from build123d import *

# Parameters (mm, degrees)
MODEL_R             = 1.2065
BOSS_EXTRUDE1_DEPTH = 6.6


with BuildPart() as part:
    # Model → Boss-Extrude1 (new body)
    with BuildSketch(Plane.XY):
        with BuildLine():
            Line((-38.1, -33.25), (-38.1, -45.95))
            ThreePointArc((-38.1, -45.95), (-37.367766953, -47.717766953), (-35.6, -48.45))
            Line((-35.6, -48.45), (10.2, -48.45))
            ThreePointArc((10.2, -48.45), (11.967766953, -47.717766953), (12.7, -45.95))
            Line((12.7, -45.95), (12.7, -3.87))
            Line((12.7, -3.87), (16.7, -3.87))
            ThreePointArc((16.7, -3.87), (18.467766953, -3.137766953), (19.2, -1.37))
            Line((19.2, -1.37), (19.2, 8.63))
            ThreePointArc((19.2, 8.63), (18.467766953, 10.397766953), (16.7, 11.13))
            Line((16.7, 11.13), (12.7, 11.13))
            Line((12.7, 11.13), (12.7, 28.25))
            ThreePointArc((12.7, 28.25), (11.967766953, 30.017766953), (10.2, 30.75))
            Line((10.2, 30.75), (-10.2, 30.75))
            ThreePointArc((-10.2, 30.75), (-11.967766953, 30.017766953), (-12.7, 28.25))
            Line((-12.7, 28.25), (-12.7, 11.13))
            Line((-12.7, 11.13), (-16.7, 11.13))
            ThreePointArc((-16.7, 11.13), (-18.467766953, 10.397766953), (-19.2, 8.63))
            Line((-19.2, 8.63), (-19.2, -1.37))
            ThreePointArc((-19.2, -1.37), (-18.467766953, -3.137766953), (-16.7, -3.87))
            Line((-16.7, -3.87), (-12.7, -3.87))
            Line((-12.7, -3.87), (-12.7, -30.75))
            Line((-12.7, -30.75), (-35.6, -30.75))
            ThreePointArc((-35.6, -30.75), (-37.367766953, -31.482233047), (-38.1, -33.25))
        make_face()
        with Locations((-33.9438, -42.1983)):
            Circle(MODEL_R, mode=Mode.SUBTRACT)
        with Locations((-24.3426, -42.1983)):
            Circle(MODEL_R, mode=Mode.SUBTRACT)
    extrude(amount=BOSS_EXTRUDE1_DEPTH)


solid = part.part
Geometry: final body of the model. Coordinates: model frame, mm. A direction names the side the tool comes from. Give positions to 0.01 mm unless a question says otherwise; leave off trailing zeros. Write each loop counter-clockwise with the first axis right and the second up, starting at its lowest first coordinate (ties: lowest second). Pieces come first, ordered by that corner, then holes. Notation, with made-up numbers: (45, -24) - (57, -24) arc R10 cw to (57, -5) - close; hole circle Ø3 at (-6.75, 3). An arc over 180 degrees is marked (long way). Return JSON: item names as keys, results as strings. Group by question number.
1) Section A-A on x = -15. Return the cut outline in (y, z).
2) First-contact query: P1, Ø3, axis at x = -4, y = -19.5, coming from the -Z side; P2, Ø2, axis at x = -15, z = 3, coming from the +Y side; P3, Ø1, axis at y = -30.5, z = 4, coming from the -X side; P4, Ø2, axis at y = 23, z = 3, coming from the +X side. Flat tips, straight axial feed; report the tip coordinate or a pass-through.
3) Mould query, pull axis Y, two halves, no side actions, for faces 5 (the cylindrical face through (18.487, 10.378, 3.254)), 6 (the flat face through (-15, -3.87, 3)), 7 (the cylindrical face through (-37.387, -47.698, 3.254)). Classes: released by +Y, released by -Y, zero draft, split by the parting line, or undercut.
4) Set-up query: faces 1 (the flat face through (-12.7, 20, 3)), 2 (the flat face through (-3, -8, 6.6)), 3 (the flat face through (15, -3.87, 3)), 4 (the cylindrical face through (-18.487, -3.118, 3.254)). Return all of +Z, -Z, +X, -X, +Y, -Y with unobstructed straight access to the full face (end or side cutting, diameter ignored); none if empty.
5) Section C-C on y = -15.5. Return the cut outline in (x, z), plus the area to 3 significant figures.
6) Line query: line 1 (Y direction, x = -17, z = 5.75); line 2 (X direction, y = 26, z = 2); line 3 (Y direction, x = -34, z = 5.25). Output: solid intervals per line, ascending.
7) Section B-B on z = 3. Return the cut outline in (x, y).
8) Section D-D on x = -28.5. Return the cut outline in (y, z).
Filled in:
{
 "1": {"outline": "(-48.45, 0) - (-30.75, 0) - (-30.75, 6.6) - (-48.45, 6.6) - close; (-3.87, 0) - (11.13, 0) - (11.13, 6.6) - (-3.87, 6.6) - close"},
 "2": {"P1": "stops at z = 0", "P2": "stops at y = 11.13", "P3": "stops at x = -36.69", "P4": "stops at x = 12.7"},
 "3": {"face 5": "released by +Y", "face 6": "undercut", "face 7": "released by -Y"},
 "4": {"face 1": "+Z, -Z, -X, +Y", "face 2": "+Z, +X, -X, +Y, -Y", "face 3": "+Z, -Z, +X, -Y", "face 4": "+Z, -Z, -X"},
 "5": {"outline": "(-12.7, 0) - (12.7, 0) - (12.7, 6.6) - (-12.7, 6.6) - close", "area": "168 mm^2"},
 "6": {"line 1": "y = -48.45 to -30.75, -3.85 to 11.11", "line 2": "x = -12.7 to 12.7", "line 3": "y = -48.45 to -43.4, -40.99 to -30.75"},
 "7": {"outline": "(-38.1, -45.95) arc R2.5 ccw to (-35.6, -48.45) - (10.2, -48.45) arc R2.5 ccw to (12.7, -45.95) - (12.7, -3.87) - (16.7, -3.87) arc R2.5 ccw to (19.2, -1.37) - (19.2, 8.63) arc R2.5 ccw to (16.7, 11.13) - (12.7, 11.13) - (12.7, 28.25) arc R2.5 ccw to (10.2, 30.75) - (-10.2, 30.75) arc R2.5 ccw to (-12.7, 28.25) - (-12.7, 11.13) - (-16.7, 11.13) arc R2.5 ccw to (-19.2, 8.63) - (-19.2, -1.37) arc R2.5 ccw to (-16.7, -3.87) - (-12.7, -3.87) - (-12.7, -30.75) - (-35.6, -30.75) arc R2.5 ccw to (-38.1, -33.25) - close; hole circle Ø2.41 at (-33.94, -42.2); hole circle Ø2.41 at (-24.34, -42.2)"},
 "8": {"outline": "(-48.45, 0) - (-30.75, 0) - (-30.75, 6.6) - (-48.45, 6.6) - close"}
}
